from build123d import *

# Parameters (mm, degrees)
EXTRUDE_THIN1_DEPTH = 698.5
FILLET1_R           = 1.27


with BuildPart() as part:
    # Sketch1 → Extrude-Thin1 (new body)
    with BuildSketch(Plane.XY):
        with BuildLine():
            Line((30.1625, 11.509375), (34.925, 11.90625))
            Line((34.925, 11.90625), (34.925, 6.35))
            Line((34.925, 6.35), (28.575, 0))
            Line((28.575, 0), (20.6375, 0))
            ThreePointArc((20.6375, 0), (19.84375, 0.79375), (19.05, 0))
            Line((19.05, 0), (-19.05, 0))
            ThreePointArc((-19.05, 0), (-19.84375, 0.79375), (-20.6375, 0))
            Line((-20.6375, 0), (-28.575, 0))
            Line((-28.575, 0), (-34.925, 6.35))
            Line((-34.925, 6.35), (-34.925, 11.90625))
            Line((-34.925, 11.90625), (-30.1625, 11.509375))
            Line((-30.1625, 11.509375), (-30.267967759, 10.243761887))
            Line((-30.267967759, 10.243761887), (-33.655, 10.526014574))
            Line((-33.655, 10.526014574), (-33.655, 6.876051224))
            Line((-33.655, 6.876051224), (-28.048948776, 1.27))
            Line((-28.048948776, 1.27), (-21.470453434, 1.27))
            ThreePointArc((-21.470453434, 1.27), (-19.84375, 2.06375), (-18.217046566, 1.27))
            Line((-18.217046566, 1.27), (18.217046566, 1.27))
            ThreePointArc((18.217046566, 1.27), (19.84375, 2.06375), (21.470453434, 1.27))
            Line((21.470453434, 1.27), (28.048948776, 1.27))
            Line((28.048948776, 1.27), (33.655, 6.876051224))
            Line((33.655, 6.876051224), (33.655, 10.526014574))
            Line((33.655, 10.526014574), (30.267967759, 10.243761887))
            Line((30.267967759, 10.243761887), (30.1625, 11.509375))
        make_face()
    extrude(amount=-EXTRUDE_THIN1_DEPTH)

    # Fillet1
    fillet1_edges = [part.edges().sort_by_distance(p)[0] for p in [
        (34.925, 11.90625, -349.25),
        (34.925, 6.35, -349.25),
        (28.575, 0, -349.25),
        (20.6375, 0, -349.25),
        (19.05, 0, -349.25),
        (-19.05, 0, -349.25),
        (-20.6375, 0, -349.25),
        (-28.575, 0, -349.25),
        (-34.925, 6.35, -349.25),
        (-34.925, 11.90625, -349.25),
    ]]
    fillet(fillet1_edges, radius=FILLET1_R)


solid = part.part
Input: part model. Units: mm. Frame: model coordinates. Round coordinates to 2 decimals unless told otherwise and drop trailing zeros. Write each loop counter-clockwise with the first axis right and the second up, starting at its lowest first coordinate (ties: lowest second). Pieces come first, ordered by that corner, then holes.
1) Cut plane B-B (x = 6.5). Return the cut outline in (y, z), then the cut area to 3 significant figures.
2) Ray query, L1, parallel to X at y = 7, z = -112 (3 decimals); L2, parallel to Y at x = -1, z = -582; L3, parallel to X at y = 3.75, z = -658 (3 decimals). Return the intervals inside material, ascending.
3) Draft query along X for faces 1 (the flat face through (3, 1, -698.5)), 2 (the flat face through (0, 1.27, -344)). Return one class per face: pulls with the +X half, pulls with the -X half, needs draft (parallel to the pull), parting line crosses it, or undercut.
4) Contact query for flat-ended pins moving along their axis: P1, Ø4, axis at y = 4.5, z = -541.5, coming from the -X side; P2, Ø5, axis at y = 6.5, z = -251, coming from the +X side (3 decimals); P3, Ø2, axis at x = -23.5, z = -401.5, coming from the +Y side; P4, Ø1.5, axis at y = 3.5, z = -462.5, coming from the -X side (3 decimals). Output: stop coordinate, or through.
Geometry says:
1. outline: (0, -698.5) - (1.27, -698.5) - (1.27, 0) - (0, 0) - close
1. area: 887 mm2
2. L1: x = -34.925 to -33.655, 33.655 to 34.925
2. L2: y = 0 to 1.27
2. L3: x = -32.325 to -30.529, 30.529 to 32.325
3. face 1: needs draft
3. face 2: undercut
4. P1: stops at x = -34.87
4. P2: stops at x = 34.925
4. P3: stops at y = 1.27
4. P4: stops at x = -32.825
